```python
from build123d import *

# Parameters (mm, degrees)
BASPROSKE_W             = 12.7
BASPROSKE_H             = 20.6375
TOOTHCUT_DEPTH          = 32.829276029
TEETHCUTS_COUNT         = 24
BORSKE_R                = 6.35
BORE_DEPTH              = 50.8000508
KEYSKE_W                = 3.175
KEYSKE_H                = 7.4676
KEYWAY_DEPTH            = 50.8000508
SKETCH1_W               = 3.175
SKETCH1_H               = 0.4064
CUT_EXTRUDE3_DEPTH      = 32.669469117
CUT_EXTRUDE3_DEPTH_BACK = 32.669469117


with BuildPart() as part:
    # BasProSke → Base-Revolve (revolve)
    with BuildSketch(Plane(origin=(0, 0, 0), x_dir=(1, 0, 0), z_dir=(0, 1, 0)), mode=Mode.PRIVATE) as base_revolve_sk:
        with Locations((6.35, 10.31875)):
            Rectangle(BASPROSKE_W, BASPROSKE_H)
    revolve(base_revolve_sk.sketch.rotate(Axis((-10, 0, 0), (1, 0, 0)), 180), axis=Axis((-10, 0, 0), (1, 0, 0)))

    # TooCutSke → ToothCut (cut, through all)
    with BuildSketch(Plane(origin=(0, 0, 0), x_dir=(0, 0, -1), z_dir=(1, 0, 0))):
        with BuildLine():
            ThreePointArc((0.762542858, 17.047308877), (0, 17.064355), (-0.762542858, 17.047308877))
            ThreePointArc((-0.762542858, 17.047308877), (-1.295412414, 18.888113288), (-2.270705673, 20.537753824))
            ThreePointArc((-2.270705673, 20.537753824), (0, 20.6629), (2.270705673, 20.537753824))
            ThreePointArc((2.270705673, 20.537753824), (1.295412414, 18.888113288), (0.762542858, 17.047308877))
        make_face()
    toothcut = extrude(amount=TOOTHCUT_DEPTH, mode=Mode.SUBTRACT)

    # TeethCuts: ToothCut ×24 about axis
    teethcuts_axis = Axis((0, 0, 0), (1, 0, 0))
    for i in range(1, TEETHCUTS_COUNT):
        add(toothcut.rotate(teethcuts_axis, i * 360 / TEETHCUTS_COUNT), mode=Mode.SUBTRACT)

    # BorSke → Bore (cut, symmetric)
    with BuildSketch(Plane(origin=(0, 0, 0), x_dir=(0, 0, -1), z_dir=(1, 0, 0))):
        with Locations(Location((0, 0, 0), (0, 0, 180))):
            Circle(BORSKE_R)
    extrude(amount=BORE_DEPTH, both=True, mode=Mode.SUBTRACT)

    # KeySke → Keyway (cut, symmetric)
    with BuildSketch(Plane(origin=(0, 0, 0), x_dir=(0, 0, -1), z_dir=(1, 0, 0))):
        with Locations((0, 3.7338)):
            Rectangle(KEYSKE_W, KEYSKE_H)
    extrude(amount=KEYWAY_DEPTH, both=True, mode=Mode.SUBTRACT)

    # Sketch1 → Cut-Extrude3 (cut, two sides)
    with BuildSketch(Plane(origin=(12.7, 0, 0), x_dir=(0, 0, -1), z_dir=(1, 0, 0))) as cut_extrude3_sk:
        with Locations((0, 7.6708)):
            Rectangle(SKETCH1_W, SKETCH1_H)
    extrude(amount=CUT_EXTRUDE3_DEPTH, mode=Mode.SUBTRACT)
    extrude(cut_extrude3_sk.sketch, amount=-CUT_EXTRUDE3_DEPTH_BACK, mode=Mode.SUBTRACT)


solid = part.part
```
Input: part model. Units: mm. Frame: model coordinates. A direction names the side the tool comes from. Round coordinates to 2 decimals unless told otherwise and drop trailing zeros. Write each loop counter-clockwise with the first axis right and the second up, starting at its lowest first coordinate (ties: lowest second). Pieces come first, ordered by that corner, then holes. Notation, with made-up numbers: M 34,-30.5 L 46,-30.5 A8 cw 46,-25.5 Z; hole C 48,12.5 d9. An arc over 180 degrees is marked long. Write each question's results on one line, items separated by ' | '.
Q1. Section query C-C (z = -10.5). Return loops of the section in (x, y), and give its area (3 significant figures).
Results:
outline: M 0,-15.66 L 12.7,-15.66 L 12.7,15.66 L 0,15.66 Z | area: 398 mm^2
Q2. Line query: line 1 along Y through (x, z) = (9.5, 0); line 2 along Z through (x, y) = (8.5, 0); line 3 along Z through (x, y) = (3.5, 12). Output: solid intervals per line, ascending.
Results:
line 1: y = -17.06 to -6.35, 7.87 to 17.06 | line 2: z = -17.06 to -6.35, 6.35 to 17.06 | line 3: z = -16.55 to -13.35, -12.13 to 12.13, 13.35 to 16.55
Q3. Section query A-A (y = 0). Return loops of the section in (x, z), and give its area (3 significant figures).
Results:
outline: M 0,-17.06 L 12.7,-17.06 L 12.7,-6.35 L 0,-6.35 Z; M 0,6.35 L 12.7,6.35 L 12.7,17.06 L 0,17.06 Z | area: 272 mm^2
Q4. Pin query (flat end, axial travel): P1, Ø2, axis at x = 6, y = 12.5, coming from the -Z side; P2, Ø1.9, axis at x = 6, y = 7, coming from the -Z side; P3, Ø4, axis at x = 4.5, y = -6, coming from the +Z side; P4, Ø10, axis at y = 0, z = 0, coming from the -X side. Return the tip coordinate at first contact, or that it passes through.
Results:
P1: stops at z = -16.64 | P2: stops at z = -19.23 | P3: stops at z = 19.23 | P4: passes through
Q5. Access query for faces 1 (the face through (6.261, 18.591, 3.636)), 2 (the face through (6.261, 15.685, 10.533)), 3 (the face through (6.26, 6.15, 17.92)), 4 (the face through (6.261, -0.011, -17.064)). Directions: +Z, -Z, +X, -X, +Y, -Y. A direction counts if a zero-diameter tool reaches every point of the face in a straight line with its end or side. Return the directions, or none.
Results:
face 1: +X, -X | face 2: +X, -X, +Y | face 3: +Z, +X, -X | face 4: -Z, +X, -X
Q6. Section query B-B (z = 0). Return loops of the section in (x, y).
Results:
outline: M 0,-17.06 L 12.7,-17.06 L 12.7,-6.35 L 0,-6.35 Z; M 0,7.87 L 12.7,7.87 L 12.7,17.06 L 0,17.06 Z
Q7. Draft query along Z for faces 5 (the face through (6.26, -16.48, 4.43)), 6 (the face through (6.26, 1.28, -18.85)), 7 (the face through (6.3, 1.3, 18.9)). Return one class per face: released by +Z, released by -Z, zero draft, split by the parting line, or undercut.
Results:
face 5: undercut | face 6: released by -Z | face 7: released by +Z
